Design review of the part built by this model. Coordinates are the model's own, in mm. A direction names the side the tool comes from. Round coordinates to 2 decimals unless told otherwise and drop trailing zeros. Write each loop counter-clockwise with the first axis right and the second up, starting at its lowest first coordinate (ties: lowest second). Pieces come first, ordered by that corner, then holes. Notation, with made-up numbers: (-16, -16.75) -> (6, -16.75) arc R29 cw to (6, 4.25) -> close; hole circle Ø11 at (37, 11.5). An arc over 180 degrees is marked (long way). Write item = value, one per line. Start each with the question number.
Item 1: Mouldability with a two-part tool opening along X and no side actions: class faces 4 (the cylindrical face through (-32.59, 2.15, 30.96)), 5 (the flat face through (15, 24, -21.25)), 6 (the flat face through (0, -11, -27.64)) as released by +X, released by -X, zero draft, split by the parting line, or undercut.
Item 2: Add section D-D, the plane x = -28. State the section outline as (y, z) points, then the cut area to 3 significant figures.
Item 3: Add section B-B, the plane y = 58. State the section outline as (x, z) points, then the cut area to 3 significant figures.
Item 4: To check wall thickness, follow L1, parallel to Z at x = 12.5, y = 39; L2, parallel to Z at x = 29, y = 38 (3 decimals); L3, parallel to Y at x = -2.5, z = -15. State the ranges of each line that lie inside material, in increasing order.
Item 5: Machinability: for faces 1 (the flat face through (-43, 3.575, 31)), 2 (the flat face through (11, 48, -22)), 3 (the flat face through (8.583, 24, -24)), which of the approach directions +Z, -Z, +X, -X, +Y, -Y give a long, thin tool a straight path to every point of the face, cutting with its end or side? Answer none if there is none.
Item 6: Add section A-A, the plane y = 38. State the section outline as (x, z) points (3 decimals), then the cut area to 3 significant figures.
Item 7: Add section C-C, the plane z = -37.64. State the section outline as (x, y) points (3 decimals), then the cut area to 3 significant figures.
Item 8: For pin 1 Ø5 at (y, z) = (45.5, 19.5) entering from -X; pin 2 Ø3 at (x, y) = (3.5, 45) entering from -Z; pin 3 Ø3.5 at (x, z) = (-41, 31) entering from -Y (3 decimals), all flat-tipped, find the tip position at first contact; note any pin that passes through.
from build123d import *

# Parameters (mm, degrees)
BOSS_EXTRUDE1_DEPTH = 48
SKETCH2_W           = 62.166
SKETCH2_H           = 62.166
BOSS_EXTRUDE2_DEPTH = 50
SKETCH5_W           = 7
SKETCH5_H           = 44.425
BOSS_EXTRUDE3_DEPTH = 20
SKETCH8_W           = 62.166
SKETCH8_H           = 7
BOSS_EXTRUDE4_DEPTH = 20
SKETCH10_W          = 7
SKETCH10_H          = 25
BOSS_EXTRUDE5_DEPTH = 20
SKETCH7_R           = 3.175
CUT_EXTRUDE1_DEPTH  = 112.997755
SKETCH9_R           = 3.175
CUT_EXTRUDE2_DEPTH  = 114.505068
SKETCH11_R          = 3.175
CUT_EXTRUDE3_DEPTH  = 114.505068
FILLET1_R           = 2
FILLET2_START       = 25.526
FILLET2_DEPTH       = 9
FILLET2_START_2     = 22.083
FILLET2_2_DEPTH     = 9
FILLET2_START_3     = -2
FILLET2_3_DEPTH     = 37


with BuildPart() as part:
    # Sketch1 → Boss-Extrude1 (new body)
    with BuildSketch(Plane(origin=(0, 0, 0), x_dir=(1, 0, 0), z_dir=(0, 1, 0))):
        Polygon((8.583, 21.25), (8.583, 27.64), (31.083, 27.64), (31.083, -34.526), (-31.083, -34.526), (-31.083, 27.64), (-8.583, 27.64), (-8.583, 21.25), (-21.25, 21.25), (-21.25, -21.25), (21.25, -21.25), (21.25, 21.25), align=None)
    extrude(amount=BOSS_EXTRUDE1_DEPTH)

    # Sketch2 → Boss-Extrude2 (add)
    with BuildSketch(Plane(origin=(0, 0, 0), x_dir=(1, 0, 0), z_dir=(0, 1, 0))):
        with Locations((0, -3.443)):
            Rectangle(SKETCH2_W, SKETCH2_H)
    extrude(amount=-BOSS_EXTRUDE2_DEPTH)

    # Sketch5 → Boss-Extrude3 (add)
    with BuildSketch(Plane(origin=(0, 0, -27.64), x_dir=(-1, 0, 0), z_dir=(0, 0, -1))):
        with Locations((-27.583, 25.7875)):
            Rectangle(SKETCH5_W, SKETCH5_H)
    extrude(amount=BOSS_EXTRUDE3_DEPTH)

    # Sketch8 → Boss-Extrude4 (add)
    with BuildSketch(Plane(origin=(0, 48, 0), x_dir=(1, 0, 0), z_dir=(0, 1, 0))):
        with Locations((0, -31.026)):
            Rectangle(SKETCH8_W, SKETCH8_H)
    extrude(amount=BOSS_EXTRUDE4_DEPTH)

    # Sketch10 → Boss-Extrude5 (add)
    with BuildSketch(Plane.ZY.offset(31.083)):
        with Locations((31.026, 16.075)):
            Rectangle(SKETCH10_W, SKETCH10_H)
    extrude(amount=BOSS_EXTRUDE5_DEPTH)

    # Sketch7 → Cut-Extrude1 (cut, through all)
    with BuildSketch(Plane.ZY.offset(-24.083)):
        with Locations(Location((-37.64, 38, 0), (0, 0, 270))):
            Circle(SKETCH7_R)
        with Locations(Location((-37.64, 18.575, 0), (0, 0, 270))):
            Circle(SKETCH7_R)
    extrude(amount=-CUT_EXTRUDE1_DEPTH, mode=Mode.SUBTRACT)

    # Sketch9 → Cut-Extrude2 (cut, through all)
    with BuildSketch(Plane(origin=(0, 0, 27.526), x_dir=(-1, 0, 0), z_dir=(0, 0, -1))):
        with Locations((-16.083, 58)):
            Circle(SKETCH9_R)
        with Locations((16.083, 58)):
            Circle(SKETCH9_R)
    extrude(amount=-CUT_EXTRUDE2_DEPTH, mode=Mode.SUBTRACT)

    # Sketch11 → Cut-Extrude3 (cut, through all)
    with BuildSketch(Plane(origin=(0, 0, 27.526), x_dir=(-1, 0, 0), z_dir=(0, 0, -1))):
        with Locations((41.083, 18.575)):
            Circle(SKETCH11_R)
    extrude(amount=-CUT_EXTRUDE3_DEPTH, mode=Mode.SUBTRACT)

    # Fillet1
    # the kernel refuses this fillet: 2 mm, written as the material it adds along each edge
    with BuildSketch(Plane(origin=(31.083, 48, 27.526), x_dir=(0, 0, -1), z_dir=(-1, 0, 0))) as fillet1_piece_1:
        with BuildLine():
            CenterArc((FILLET1_R, -FILLET1_R), FILLET1_R, 90, 90)
            Line((0, -FILLET1_R), (0, 0))
            Line((0, 0), (FILLET1_R, 0))
        make_face()
    extrude(amount=62.166)
    with BuildSketch(Plane(origin=(-31.083, 28.575, 27.526), x_dir=(0, 0, -1), z_dir=(0, -1, 0))) as fillet1_piece_2:
        with BuildLine():
            CenterArc((FILLET1_R, -FILLET1_R), FILLET1_R, 90, 90)
            Line((0, -FILLET1_R), (0, 0))
            Line((0, 0), (FILLET1_R, 0))
        make_face()
    extrude(amount=25)
    with BuildSketch(Plane(origin=(24.083, 48, -27.64), x_dir=(-1, 0, 0), z_dir=(0, -1, 0))) as fillet1_piece_3:
        with BuildLine():
            CenterArc((FILLET1_R, FILLET1_R), FILLET1_R, 180, 90)
            Line((0, FILLET1_R), (0, 0))
            Line((0, 0), (FILLET1_R, 0))
        make_face()
    extrude(amount=44.425)

    # Fillet2: read off the stored shape, not the designer's step
    # Fillet2 outline → Fillet2 (add)
    with BuildSketch(Plane.XY.offset(FILLET2_START)):
        with BuildLine():
            Line((-31.083, -1.425), (-31.083, 3.575))
            Line((-31.083, 3.575), (-36.083, 3.575))
            ThreePointArc((-36.083, 3.575), (-32.547466, 2.110534), (-31.083, -1.425))
        make_face()
        with BuildLine():
            ThreePointArc((-31.083, 33.575), (-32.547466, 30.039466), (-36.083, 28.575))
            Line((-36.083, 28.575), (-31.083, 28.575))
            Line((-31.083, 28.575), (-31.083, 33.575))
        make_face()
    extrude(amount=FILLET2_DEPTH)

    # Fillet2 2 outline → Fillet2 2 (add)
    with BuildSketch(Plane.YZ.offset(FILLET2_START_2)):
        with BuildLine():
            ThreePointArc((-1.425, -27.64), (2.110534, -29.104466), (3.575, -32.64))
            Line((3.575, -32.64), (3.575, -27.64))
            Line((3.575, -27.64), (-1.425, -27.64))
        make_face()
    extrude(amount=FILLET2_2_DEPTH)

    # Fillet2 3 outline → Fillet2 3 (cut)
    with BuildSketch(Plane(origin=(0, 0, 0), x_dir=(1, 0, 0), z_dir=(0, 1, 0)).offset(FILLET2_START_3)):
        with BuildLine():
            ThreePointArc((-33.083, -27.526), (-31.668786, -26.940214), (-31.083, -25.526))
            Line((-31.083, -25.526), (-36.083, -25.526))
            Line((-36.083, -25.526), (-36.083, -27.526))
            Line((-36.083, -27.526), (-33.083, -27.526))
        make_face()
        with BuildLine():
            Line((24.083, 32.64), (22.083, 32.64))
            Line((22.083, 32.64), (22.083, 27.64))
            ThreePointArc((22.083, 27.64), (23.497214, 28.225786), (24.083, 29.64))
            Line((24.083, 29.64), (24.083, 32.64))
        make_face()
    extrude(amount=FILLET2_3_DEPTH, mode=Mode.SUBTRACT)


solid = part.part
Result set:
q1.face_4 = released by -X
q1.face_5 = undercut
q1.face_6 = zero draft
q2.outline = (-50, -27.64) -> (48, -27.64) -> (48, 25.53) arc R2 cw to (50, 27.53) -> (68, 27.53) -> (68, 34.53) -> (-50, 34.53) -> close
q2.area = 6,230 mm²
q3.outline = (-31.08, 27.53) -> (-19.26, 27.53) -> (-19.26, 34.53) -> (-31.08, 34.53) -> close; (-12.91, 27.53) -> (12.91, 27.53) -> (12.91, 34.53) -> (-12.91, 34.53) -> close; (19.26, 27.53) -> (31.08, 27.53) -> (31.08, 34.53) -> (19.26, 34.53) -> close
q3.area = 346 mm²
q4.L1 = -27.64 to -21.25, 21.25 to 34.53
q4.L2 = -47.64 to -40.815, -34.465 to 34.526
q4.L3 = -50 to 0
q5.face_1 = +Z, -Z, -X, -Y
q5.face_2 = -Z, +X, -X, +Y
q5.face_3 = -Z, +Y
q6.outline = (-31.083, -27.64) -> (-8.583, -27.64) -> (-8.583, -21.25) -> (-21.25, -21.25) -> (-21.25, 21.25) -> (21.25, 21.25) -> (21.25, -21.25) -> (8.583, -21.25) -> (8.583, -27.64) -> (22.083, -27.64) arc R2 cw to (24.083, -29.64) -> (24.083, -34.465) -> (31.083, -34.465) -> (31.083, 34.526) -> (-31.083, 34.526) -> close; (24.083, -47.64) -> (31.083, -47.64) -> (31.083, -40.815) -> (24.083, -40.815) -> close
q6.area = 2,050 mm²
q7.outline = (24.083, 3.575) -> (31.083, 3.575) -> (31.083, 15.4) -> (24.083, 15.4) -> close; (24.083, 21.75) -> (31.083, 21.75) -> (31.083, 34.825) -> (24.083, 34.825) -> close; (24.083, 41.175) -> (31.083, 41.175) -> (31.083, 48) -> (24.083, 48) -> close
q7.area = 222 mm²
q8.pin_1 = -31.08
q8.pin_2 = 21.25
q8.pin_3 = 3.575
